from build123d import *

# Parameters (mm, degrees)
BOSS_EXTRUDE1_DEPTH = 284
CUT_EXTRUDE1_DEPTH  = 336.560724758
CUT_EXTRUDE3_DEPTH  = 284
SKETCH5_W           = 284
SKETCH5_H           = 2
BOSS_EXTRUDE2_DEPTH = 5
SKETCH6_W           = 284
SKETCH6_H           = 2
BOSS_EXTRUDE3_DEPTH = 5


with BuildPart() as part:
    # Sketch1 → Boss-Extrude1 (new body)
    with BuildSketch(Plane.XY):
        with BuildLine():
            Line((50, 1), (52, 1))
            Line((52, 1), (52, -1))
            Line((52, -1), (-52, -1))
            Line((-52, -1), (-52, 1))
            Line((-52, 1), (-50, 1))
            ThreePointArc((-50, 1), (-48.585786438, 1.585786438), (-48, 3))
            Line((-48, 3), (-48, 169))
            ThreePointArc((-48, 169), (-47.414213562, 170.414213562), (-46, 171))
            Line((-46, 171), (46, 171))
            ThreePointArc((46, 171), (47.414213562, 170.414213562), (48, 169))
            Line((48, 169), (48, 3))
            ThreePointArc((48, 3), (48.585786438, 1.585786438), (50, 1))
        make_face()
    extrude(amount=BOSS_EXTRUDE1_DEPTH)

    # Sketch2 → Cut-Extrude1 (cut, through all)
    with BuildSketch(Plane(origin=(0, 0, 0), x_dir=(-1, 0, 0), z_dir=(0, 0, -1))):
        with BuildLine():
            Line((-46.535898385, 1), (46.535898385, 1))
            ThreePointArc((46.535898385, 1), (46.136296695, 1.96472382), (46, 3))
            Line((46, 3), (46, 169))
            Line((46, 169), (-46, 169))
            Line((-46, 169), (-46, 3))
            ThreePointArc((-46, 3), (-46.136296695, 1.96472382), (-46.535898385, 1))
        make_face()
    extrude(amount=-CUT_EXTRUDE1_DEPTH, mode=Mode.SUBTRACT)

    # Sketch3 → Cut-Extrude3 (cut)
    with BuildSketch(Plane(origin=(0, 0, 0), x_dir=(-1, 0, 0), z_dir=(0, 0, -1))):
        with BuildLine():
            Line((-50.018137883, -1.031749995), (49.461412471, -2.32808526))
            ThreePointArc((49.461412471, -2.32808526), (47.495708501, -1.106152193), (46.535898385, 1))
            Line((46.535898385, 1), (-46.535898385, 1))
            ThreePointArc((-46.535898385, 1), (-48.002325394, -0.486674019), (-50.018137883, -1.031749995))
        make_face()
    extrude(amount=-CUT_EXTRUDE3_DEPTH, mode=Mode.SUBTRACT)

    # Sketch5 → Boss-Extrude2 (add)
    with BuildSketch(Plane.ZY.offset(52)):
        with Locations((142, 0)):
            Rectangle(SKETCH5_W, SKETCH5_H)
    extrude(amount=BOSS_EXTRUDE2_DEPTH)

    # Sketch6 → Boss-Extrude3 (add)
    with BuildSketch(Plane(origin=(52, 0, 0), x_dir=(0, 0, -1), z_dir=(1, 0, 0))):
        with Locations((-142, 0)):
            Rectangle(SKETCH6_W, SKETCH6_H)
    extrude(amount=BOSS_EXTRUDE3_DEPTH)


solid = part.part
Work out the finished part from the listing and answer in its coordinate system (mm). A direction names the side the tool comes from. Coordinates: 2 decimals unless noted, no trailing zeros. Write each loop counter-clockwise with the first axis right and the second up, starting at its lowest first coordinate (ties: lowest second). Pieces come first, ordered by that corner, then holes. Notation, with made-up numbers: (-36.75, -40) - (10.25, -40) arc R7 cw to (10.25, -32) - close; hole circle Ø9 at (-32.75, 39.5). An arc over 180 degrees is marked (long way). One line per question, with ' | ' between items.
1) The mould has two halves that part along X. Classify faces 1 (the face through (-1, 169, 140)), 2 (the face through (53, -1, 144)), 3 (the face through (-48, 85, 140)): +X half, -X half, draft (parallel to the pull), parting line (faces both ways), or undercut.
Checks:
face 1: undercut | face 2: draft | face 3: -X half
2) Find section B-B, the plane z = 30.5. Determine the outline of the cut face in (x, y).
Checks:
outline: (-57, -1) - (-47.41, -1) arc R4 ccw to (-46.54, 1) arc R4 ccw to (-46, 3) - (-46, 169) - (46, 169) - (46, 3) arc R4 ccw to (46.54, 1) arc R4 ccw to (49.52, -1) - (57, -1) - (57, 1) - (50, 1) arc R2 cw to (48, 3) - (48, 169) arc R2 ccw to (46, 171) - (-46, 171) arc R2 ccw to (-48, 169) - (-48, 3) arc R2 cw to (-50, 1) - (-57, 1) - close
3) Consider probe 1 along X at (y, z) = (117, 268.5); probe 2 along Y at (x, z) = (-37.5, 135); probe 3 along Y at (x, z) = (49.5, 134.5). Determine where each line is inside the solid, lowest interval first. Write a range as [from, to].
Checks:
probe 1: [-48, -46], [46, 48] | probe 2: [169, 171] | probe 3: [-1, 1.06]
4) Find section A-A, the plane y = 125. Determine the outline of the cut face in (x, z), and give its area (3 significant figures).
Checks:
outline: (-48, 0) - (-46, 0) - (-46, 284) - (-48, 284) - close; (46, 0) - (48, 0) - (48, 284) - (46, 284) - close | area: 1,140 mm2
5) Find section C-C, the plane x = -10. Determine the outline of the cut face in (y, z), and give its area (3 significant figures).
Checks:
outline: (169, 0) - (171, 0) - (171, 284) - (169, 284) - close | area: 568 mm2
6) Flat-ended cylindrical pins translate along their axes: P1, Ø5, axis at x = 18, z = 237.5, coming from the -Y side; P2, Ø3.5, axis at x = 53, z = 73, coming from the +Y side; P3, Ø12, axis at y = 72.5, z = 182.5, coming from the +X side. Find the tip coordinate at first contact, or state that the pin passes through.
Checks:
P1: y = 169 | P2: y = 1 | P3: x = 48
7) For faces 4 (the face through (-53, 1, 140)), 5 (the face through (48, 87, 140)), 6 (the face through (-52, -1, 140)), 7 (the face through (46, 87, 140)), determine the directions among +Z, -Z, +X, -X, +Y, -Y from which every point of the face is accessible in a straight line to the end or side of a thin tool.
Checks:
face 4: +Z, -Z, -X, +Y | face 5: +Z, -Z, +X, +Y | face 6: +Z, -Z, +X, -X, -Y | face 7: +Z, -Z, -Y
